Check sheet for the drawn part. Datum: minimum x, y, z corner. Units: mm. Coordinates: 2 decimals unless noted, no trailing zeros. Loops run counter-clockwise (first coordinate to the right, second up) from the corner with the lowest first, then second, coordinate; pieces in that order, holes last.
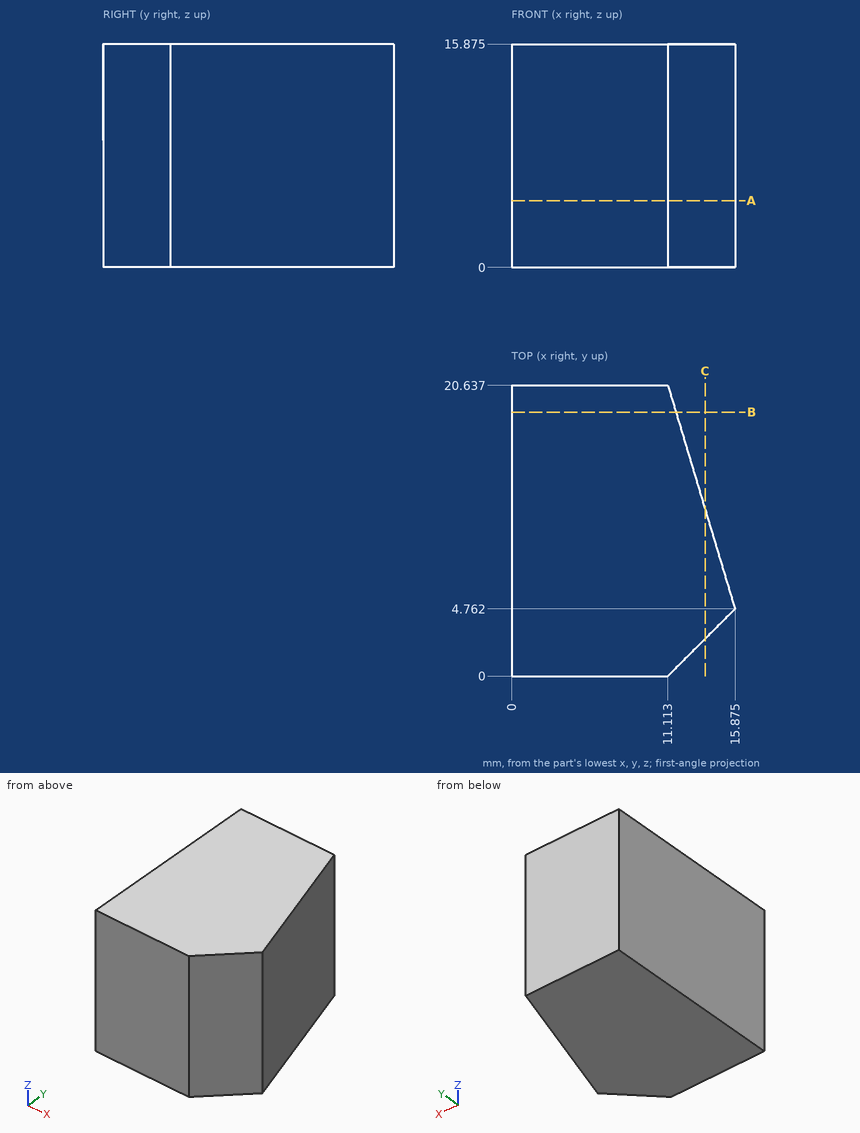
(1) Sectioned sample at B-B on y = 18.75. Record the cut outline in (x, z) (1 decimal).
Findings:
outline: (0, 0) - (11.7, 0) - (11.7, 15.9) - (0, 15.9) - close
(2) Gauge pin test, flat ends, axial feed: pin 1 Ø5 at (y, z) = (4.5, 8.5) entering from -X; pin 2 Ø1 at (y, z) = (5.5, 3.5) entering from +X. Record the tip position at first contact, or that the pin passes through.
Findings:
pin 1: stops at x = 0
pin 2: stops at x = 15.8
(3) Sectioned sample at C-C on x = 13.75. Record the cut outline in (y, z) (1 decimal).
Findings:
outline: (2.6, 0) - (11.8, 0) - (11.8, 15.9) - (2.6, 15.9) - close
(4) Scan lines: L1, parallel to X at y = 7.75, z = 8.5; L2, parallel to X at y = 14, z = 7.5 (1 decimal). Record each from-to range of solid material in increasing order.
Findings:
L1: x = 0 to 14.98
L2: x = 0 to 13.1
(5) Sectioned sample at A-A on z = 4.75. Record the cut outline in (x, y) (1 decimal).
Findings:
outline: (0, 0) - (11.1, 0) - (15.9, 4.8) - (11.1, 20.6) - (0, 20.6) - close
